CAD build for the part. Positions are in the model's coordinates, mm. A direction names the side the tool comes from. Coordinates: 2 decimals unless noted, no trailing zeros. Loops run counter-clockwise (first coordinate to the right, second up) from the corner with the lowest first, then second, coordinate; pieces in that order, holes last. Notation, with made-up numbers: (-15.5, 67) - (40.5, 67) arc R32 ccw to (40.5, 101) - close; hole circle Ø10 at (78, 2.5). An arc over 180 degrees is marked (long way). Put each result on its own line as item: value.
```python
from build123d import *

# Parameters (mm, degrees)
SKETCH1_R               = 30
SKETCH1_R_2             = 20
BOSS_EXTRUDE1_DEPTH     = 10
SKETCH2_OUTSIDE_W       = 79.436
SKETCH2_OUTSIDE_H       = 79.436
SKETCH2_OUTSIDE_R       = 20
CUT_EXTRUDE1_DEPTH      = 3.5
CUT_EXTRUDE2_DEPTH      = 44.588989435
CUT_EXTRUDE2_DEPTH_BACK = 44.588989435
SKETCH3_R               = 1.6
CUT_EXTRUDE3_DEPTH      = 47.904157598
CUT_EXTRUDE3_DEPTH_BACK = 47.904157598


with BuildPart() as part:
    # Sketch1 → Boss-Extrude1 (new, symmetric)
    # profile 1 of 2: a face of its own
    with BuildSketch(Plane.XY):
        Circle(SKETCH1_R)
        Circle(SKETCH1_R_2, mode=Mode.SUBTRACT)
    # profile 2 of 2: a face of its own
    with BuildSketch(Plane.XY):
        Circle(SKETCH1_R_2)
    extrude(amount=BOSS_EXTRUDE1_DEPTH, both=True)

    # Sketch2 outside → Cut-Extrude1 (cut, symmetric)
    with BuildSketch(Plane.XY.offset(5)):
        Rectangle(SKETCH2_OUTSIDE_W, SKETCH2_OUTSIDE_H)
        Circle(SKETCH2_OUTSIDE_R, mode=Mode.SUBTRACT)
    cut_extrude1 = extrude(amount=CUT_EXTRUDE1_DEPTH, both=True, mode=Mode.SUBTRACT)

    # Mirror1: Cut-Extrude1 across plane
    add(cut_extrude1.mirror(Plane.XY), mode=Mode.SUBTRACT)

    # Sketch3 → Cut-Extrude2 (cut, two sides: drawn at the far end of the back side and taken through both)
    with BuildSketch(Plane(origin=(0, 0, 0), x_dir=(0, 0, -1), z_dir=(1, 0, 0)).offset(-CUT_EXTRUDE2_DEPTH_BACK)):
        with Locations((-5, 10)):
            Circle(SKETCH3_R)
        with Locations((5, 10)):
            Circle(SKETCH3_R)
    extrude(amount=CUT_EXTRUDE2_DEPTH + CUT_EXTRUDE2_DEPTH_BACK, mode=Mode.SUBTRACT)

    # Sketch4 → Cut-Extrude3 (cut, two sides: drawn at the far end of the back side and taken through both)
    with BuildSketch(Plane(origin=(0, 0, -10), x_dir=(-1, 0, 0), z_dir=(0, 0, -1)).offset(-CUT_EXTRUDE3_DEPTH_BACK)):
        with BuildLine():
            Line((-1.774823935, 1.9), (1.774823935, 1.9))
            ThreePointArc((1.774823935, 1.9), (0, -2.6), (-1.774823935, 1.9))
        make_face()
    extrude(amount=CUT_EXTRUDE3_DEPTH + CUT_EXTRUDE3_DEPTH_BACK, mode=Mode.SUBTRACT)


solid = part.part
```
Q1. Tool access for faces 4 (the cylindrical face through (-29.97, 1.32, 9.26)), 5 (the flat face through (6, -20, 8.5)): list every direction of +Z, -Z, +X, -X, +Y, -Y with a clear straight run to the whole face (end or side of a thin tool).
Determined:
face 4: +Z, -Z
face 5: none
Q2. Pin check, flat tips, straight feed: pin 1 Ø10 at (x, z) = (-23, -6) entering from -Y; pin 2 Ø10 at (x, z) = (2.5, 3.5) entering from +Y; pin 3 Ø1.5 at (y, z) = (1.5, 6.5) entering from -X. Stop position of each tip, or through.
Determined:
pin 1: y = -23.48
pin 2: y = 30
pin 3: x = -19.99
Q3. Slice it at A-A, the plane y = -24. Give the cut face in (x, z), then the cut area to 3 significant figures.
Determined:
outline: (-18, -10) - (18, -10) - (18, -8.5) - (-18, -8.5) - close; (-18, -1.5) - (18, -1.5) - (18, 1.5) - (-18, 1.5) - close; (-18, 8.5) - (18, 8.5) - (18, 10) - (-18, 10) - close
area: 216 mm2
Q4. Wall check: L1, parallel to Z at x = -9, y = 10; L2, parallel to Z at x = 7, y = -24.5; L3, parallel to X at y = -2, z = 0.75. Give the ranges that are in metal, low to high. Write a range as from..to.
Determined:
L1: -10..-6.6, -3.4..3.4, 6.6..10
L2: -10..-8.5, -1.5..1.5, 8.5..10
L3: -29.93..-1.66, 1.66..29.93
Q5. Slice it at D-D, the plane z = 7.75. Give the cut face in (x, y), then the cut area to 3 significant figures.
Determined:
outline: circle Ø40 at (0, 0); hole (-1.77, 1.9) arc R2.6 ccw (long way) to (1.77, 1.9) - close
area: 1,240 mm2
Q6. Slice it at C-C, the plane y = 0. Give the cut face in (x, z).
Determined:
outline: (-30, -10) - (-2.6, -10) - (-2.6, 10) - (-30, 10) - (-30, 8.5) - (-20, 8.5) - (-20, 1.5) - (-30, 1.5) - (-30, -1.5) - (-20, -1.5) - (-20, -8.5) - (-30, -8.5) - close; (2.6, -10) - (30, -10) - (30, -8.5) - (20, -8.5) - (20, -1.5) - (30, -1.5) - (30, 1.5) - (20, 1.5) - (20, 8.5) - (30, 8.5) - (30, 10) - (2.6, 10) - close
Q7. Slice it at B-B, the plane x = 0. Give the cut face in (y, z).
Determined:
outline: (-30, -10) - (-2.6, -10) - (-2.6, 10) - (-30, 10) - (-30, 8.5) - (-20, 8.5) - (-20, 1.5) - (-30, 1.5) - (-30, -1.5) - (-20, -1.5) - (-20, -8.5) - (-30, -8.5) - close; (1.9, -10) - (30, -10) - (30, -8.5) - (20, -8.5) - (20, -1.5) - (30, -1.5) - (30, 1.5) - (20, 1.5) - (20, 8.5) - (30, 8.5) - (30, 10) - (1.9, 10) - close; hole circle Ø3.2 at (10, -5); hole circle Ø3.2 at (10, 5)
Q8. Mould opens along X. For faces 1 (the flat face through (6, -20, -1.5)), 2 (the flat face through (0, 1.9, 0)), 3 (the cylindrical face through (-29.97, 1.32, 0.02)) say: +X half, -X half, draft (parallel to the pull), parting line (faces both ways), or undercut.
Determined:
face 1: draft
face 2: undercut
face 3: parting line
